Here's how the part is built. I have some questions about the finished solid (model axes, mm). Round coordinates to 2 decimals unless told otherwise and drop trailing zeros. Answer as a JSON object with one key per item and string values.
from build123d import *

# Parameters (mm, degrees)
F1_DEPTH = 19.05
F3_D     = 9.525
F4_R     = 5.08


with BuildPart() as f1:
    # F0 (on Top) → F1 (new body)
    with BuildSketch(Plane.XY):
        with BuildLine():
            Line((0, 88.9), (0, 0))
            Line((0, 0), (203.2, 0))
            ThreePointArc((203.2, 0), (248.003873, 37.392253), (304.8, 50.8))
            Line((304.8, 50.8), (965.2, 50.8))
            ThreePointArc((965.2, 50.8), (1021.996127, 37.392253), (1066.8, 0))
            Line((1066.8, 0), (1270, 0))
            Line((1270, 0), (1270, 88.9))
            Line((1270, 88.9), (0, 88.9))
        make_face()
    extrude(amount=F1_DEPTH)

    # F3 (through all)
    with Locations(Plane.XZ):
        with Locations((31.75, 9.525), (425.45, 9.525), (844.55, 9.525), (1238.25, 9.525)):
            Hole(F3_D / 2)

    # F4
    f4_edges = [f1.edges().sort_by_distance(p)[0] for p in [
        (203.2, 0, 9.525),
        (1066.8, 0, 9.525),
    ]]
    fillet(f4_edges, radius=F4_R)


solid = f1.part
Item 1: I'm going to push flat-ended pins straight in: pin 1 Ø10 at (x, z) = (999.5, 3) entering from -Y; pin 2 Ø5.5 at (x, z) = (666.5, 13.5) entering from -Y; pin 3 Ø5.5 at (x, z) = (844.55, 9.525) entering from +Y. Where does each tip first touch, or does it pass through?
Resolved:
{"pin 1": "y = 44.57", "pin 2": "y = 50.8", "pin 3": "through"}
Item 2: Please list where these lines run through material, in increasing order: probe 1 along X at (y, z) = (31, 13); probe 2 along Z at (x, y) = (31.75, 38); probe 3 along X at (y, z) = (59, 11.75). Write a range as from..to.
Resolved:
{"probe 1": "0..28.49, 35.01..236.7, 1033.3..1234.99, 1241.51..1270", "probe 2": "0..4.76, 14.29..19.05", "probe 3": "0..27.54, 35.96..421.24, 429.66..840.34, 848.76..1234.04, 1242.46..1270"}
Item 3: If we mould it in two halves opening along X, with no side actions, what happens to faces 1 (the face through (626, 55, 0)), 2 (the face through (1020.167, 38.289, 9.392)), 3 (the face through (248.38, 37.58, 9.39))? For each: pulls with the +X half, pulls with the -X half, needs draft (parallel to the pull), parting line crosses it, or undercut.
Resolved:
{"face 1": "needs draft", "face 2": "undercut", "face 3": "undercut"}
Item 4: I want a section at A-A, the plane y = 18. State how many separate pieces and enclosed holes the cut face has, then the cut area to 3 significant figures.
Resolved:
{"separate pieces": "2", "enclosed holes": "2", "area": "8,230 mm²"}
